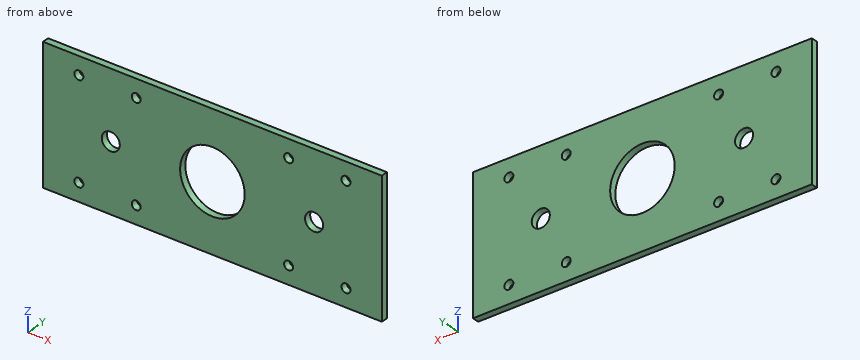
```python
from build123d import *

# Parameters (mm, degrees)
SKETCH1_W           = 150
SKETCH1_H           = 60
BOSS_EXTRUDE1_DEPTH = 3
SKETCH2_R           = 14.2875
SKETCH2_R_2         = 1.984375
SKETCH2_R_3         = 4
CUT_EXTRUDE2_DEPTH  = 4


with BuildPart() as part:
    # Sketch1 → Boss-Extrude1 (new body)
    with BuildSketch(Plane(origin=(0, 0, 0), x_dir=(1, 0, 0), z_dir=(0, 1, 0))):
        Rectangle(SKETCH1_W, SKETCH1_H)
    extrude(amount=BOSS_EXTRUDE1_DEPTH)

    # Sketch2 → Cut-Extrude2 (cut, through all)
    with BuildSketch(Plane(origin=(0, 3, 0), x_dir=(1, 0, 0), z_dir=(0, 1, 0))):
        Circle(SKETCH2_R)
        with Locations((59.125, 22.0625)):
            Circle(SKETCH2_R_2)
        with Locations((33.725, 22.0625)):
            Circle(SKETCH2_R_2)
        with Locations((33.725, -22.0625)):
            Circle(SKETCH2_R_2)
        with Locations((59.125, -22.0625)):
            Circle(SKETCH2_R_2)
        with Locations((-33.725, 22.0625)):
            Circle(SKETCH2_R_2)
        with Locations((-59.125, 22.0625)):
            Circle(SKETCH2_R_2)
        with Locations((-59.125, -22.0625)):
            Circle(SKETCH2_R_2)
        with Locations((-33.725, -22.0625)):
            Circle(SKETCH2_R_2)
        with Locations((45, 0)):
            Circle(SKETCH2_R_3)
        with Locations((-45, 0)):
            Circle(SKETCH2_R_3)
    extrude(amount=-CUT_EXTRUDE2_DEPTH, mode=Mode.SUBTRACT)


solid = part.part
```
Could you check a few things on this model? Use its own coordinates, in mm. Round coordinates to 2 decimals unless told otherwise and drop trailing zeros. Order: outer loops, then holes, each group sorted by start corner. A loop starts at its lowest first (then second) coordinate and runs counter-clockwise, first axis right, second up. Notation, with made-up numbers: M 42,48.25 L 81,48.25 A22 cw 81,66.25 Z; hole C 18.25,24 d3. An arc over 180 degrees is marked long. One line per question, with ' | ' between items. Start each with the question number.
(1) Suppose I cut it at C-C on y = 0.6. Count the separate pieces of the cut face and the enclosed holes in it, then the cut area to 3 significant figures.
(2) Suppose I cut it at A-A on x = 0. List the corners of the cut face in (y, z) for me.
(3) Please list where these lines run through material, in increasing order: line 1 along X through (y, z) = (1.95, 0); line 2 along X through (y, z) = (2.5, -22); line 3 along X through (y, z) = (1.9, 21.5).
(4) Suppose I cut it at B-B on z = 0. List the corners of the cut face in (x, y) for me.
Geometry results:
1) separate pieces: 1 | enclosed holes: 11 | area: 8,160 mm²
2) outline: M 0,-30 L 3,-30 L 3,-14.29 L 0,-14.29 Z; M 0,14.29 L 3,14.29 L 3,30 L 0,30 Z
3) line 1: -75 to -49, -41 to -14.29, 14.29 to 41, 49 to 75 | line 2: -75 to -61.11, -57.14 to -35.71, -31.74 to 31.74, 35.71 to 57.14, 61.11 to 75 | line 3: -75 to -61.03, -57.22 to -35.63, -31.82 to 31.82, 35.63 to 57.22, 61.03 to 75
4) outline: M -75,0 L -49,0 L -49,3 L -75,3 Z; M -41,0 L -14.29,0 L -14.29,3 L -41,3 Z; M 14.29,0 L 41,0 L 41,3 L 14.29,3 Z; M 49,0 L 75,0 L 75,3 L 49,3 Z
